Model file for the job. Use its own axes, mm. Face numbers are marked on the shaded views. A direction names the side the tool comes from. Give positions to 0.01 mm unless a question says otherwise; leave off trailing zeros. Order: outer loops, then holes, each group sorted by start corner. A loop starts at its lowest first (then second) coordinate and runs counter-clockwise, first axis right, second up. Notation, with made-up numbers: M 55.25,-28 L 103.25,-28 A30 ccw 103.25,-4 Z; hole C -36.75,42.25 d2. An arc over 180 degrees is marked long. Return JSON: item names as keys, results as strings. Group by question number.
1. Wall check: probe 1 along Y at (x, z) = (23.5, 6.75); probe 2 along Y at (x, z) = (102, 4.5); probe 3 along Y at (x, z) = (85, 5.25). Give the ranges that are in metal, low to high. Write a range as [from, to].
2. 3-axis set-ups, long thin cutter, end or side, ignore diameter. For the marked faces 4, 5 and 6: which of +Z, -Z, +X, -X, +Y, -Y reach the whole face in a straight line?
3. Pin check, flat tips, straight feed: pin 1 (15 mm diameter, centred on x = 26.5, y = 30.5, fed in from -Z) (3 decimals); pin 2 (2 mm diameter, centred on y = 60, z = 21, fed in from +X); pin 3 (5 mm diameter, centred on x = 111, y = 57, fed in from +Z). Stop position of each tip, or through.
4. Slice it at D-D on y = 16.5. List the corners of the cut face in (x, z) (3 decimals).
5. Slice it at B-B on y = 33.5. List the corners of the cut face in (x, z) (3 decimals), then the cut area to 3 significant figures.
6. Two-plate mould, pull along Y, no slides. Class the marked faces 1, 2 and 3: released by +Y, released by -Y, zero draft, split by the parting line, or undercut.
7. Slice it at C-C on x = 27.5. List the corners of the cut face in (y, z) (3 decimals).
8. Slice it at A-A on z = 5.5. List the corners of the cut face in (x, y) (3 decimals).
from build123d import *

# Parameters (mm, degrees)
F1_DEPTH = 22.225
F3_DEPTH = 19.685
F5_DEPTH = 19.685
F6_R     = 21
F6_R_2   = 18.75
F7_DEPTH = 7
F8_R     = 1.2446
F9_DEPTH = 2.541


with BuildPart() as f1:
    # F0 (on Top) → F1 (new body)
    with BuildSketch(Plane.XY):
        with BuildLine():
            ThreePointArc((0, 3.175), (0.929936, 0.929936), (3.175, 0))
            Line((3.175, 0), (88.9, 0))
            Line((88.9, 0), (88.9, 29.21))
            ThreePointArc((88.9, 29.21), (73.66, 44.45), (88.9, 59.69))
            Line((88.9, 59.69), (88.9, 88.9))
            Line((88.9, 88.9), (3.175, 88.9))
            ThreePointArc((3.175, 88.9), (0.929936, 87.970064), (0, 85.725))
            Line((0, 85.725), (0, 3.175))
        make_face()
        with BuildLine():
            Line((88.9, 29.21), (88.9, 0))
            ThreePointArc((88.9, 0), (133.35, 44.45), (88.9, 88.9))
            Line((88.9, 88.9), (88.9, 59.69))
            ThreePointArc((88.9, 59.69), (99.676307, 55.226307), (104.14, 44.45))
            ThreePointArc((104.14, 44.45), (99.676307, 33.673693), (88.9, 29.21))
        make_face()
    extrude(amount=F1_DEPTH)

    # F2 (on face) → F3 (cut)
    with BuildSketch(Plane.XY.offset(22.225)):
        with BuildLine():
            Line((88.9, 86.36), (88.9, 2.54))
            ThreePointArc((88.9, 2.54), (130.81, 44.45), (88.9, 86.36))
        make_face()
        with BuildLine():
            Line((56.642, 2.54), (88.9, 2.54))
            Line((88.9, 2.54), (88.9, 86.36))
            Line((88.9, 86.36), (56.642, 86.36))
            ThreePointArc((56.642, 86.36), (49.817005, 83.532995), (46.99, 76.708))
            Line((46.99, 76.708), (46.99, 12.192))
            ThreePointArc((46.99, 12.192), (49.817005, 5.367005), (56.642, 2.54))
        make_face()
    extrude(amount=-F3_DEPTH, mode=Mode.SUBTRACT)

    # F4 (on face) → F5 (cut)
    with BuildSketch(Plane(origin=(0, 0, 0), x_dir=(1, 0, 0), z_dir=(0, 0, -1))):
        with BuildLine():
            ThreePointArc((56.204695, -70.669557), (46.99, -44.45), (56.204695, -18.230443))
            ThreePointArc((56.204695, -18.230443), (57.376711, -8.015994), (48.674868, -2.54))
            Line((48.674868, -2.54), (2.54, -2.54))
            Line((2.54, -2.54), (2.54, -86.36))
            Line((2.54, -86.36), (48.674868, -86.36))
            ThreePointArc((48.674868, -86.36), (57.376711, -80.884006), (56.204695, -70.669557))
        make_face()
    extrude(amount=-F5_DEPTH, mode=Mode.SUBTRACT)

    # F6 (on face) → F7 (join)
    with BuildSketch(Plane.XY.offset(2.54)):
        with Locations((88.9, 44.45)):
            Circle(F6_R)
        with Locations((88.9, 44.45)):
            Circle(F6_R_2, mode=Mode.SUBTRACT)
    extrude(amount=F7_DEPTH)

    # F8 (on face) → F9 (cut, through all)
    with BuildSketch(Plane(origin=(0, 0, 19.685), x_dir=(1, 0, 0), z_dir=(0, 0, -1))):
        with Locations((10.1092, -43.18)):
            Circle(F8_R)
        with Locations((14.6304, -6.5786)):
            Circle(F8_R)
        with Locations((41.1226, -22.1996)):
            Circle(F8_R)
    extrude(amount=-F9_DEPTH, mode=Mode.SUBTRACT)


solid = f1.part
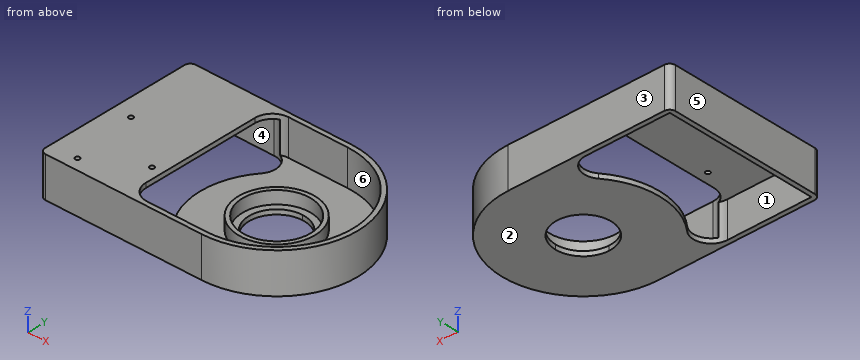
Result:
{
 "1": {"probe 1": "y = [0, 2.54], [86.36, 88.9]", "probe 2": "y = [1.97, 4.64], [28.04, 31.04], [57.86, 60.86], [84.26, 86.93]", "probe 3": "y = [0, 2.54], [23.82, 26.11], [62.79, 65.08], [86.36, 88.9]"},
 "2": {"face 4": "-Z", "face 5": "+Z, -Z, -X, +Y, -Y", "face 6": "+Z"},
 "3": {"pin 1": "stops at z = 19.685", "pin 2": "stops at x = 130.9", "pin 3": "stops at z = 2.54"},
 "4": {"outline": "M 0,0 L 2.54,0 L 2.54,19.685 L 46.99,19.685 L 46.99,22.225 L 0,22.225 Z; M 57.312,0 L 123.463,0 L 123.463,22.225 L 120.129,22.225 L 120.129,2.54 L 57.312,2.54 Z"},
 "5": {"outline": "M 0,0 L 2.54,0 L 2.54,19.685 L 46.99,19.685 L 46.99,22.225 L 0,22.225 Z; M 48.446,0 L 78.3,0 L 78.3,2.54 L 73.68,2.54 L 73.68,9.54 L 70.981,9.54 L 70.981,2.54 L 48.446,2.54 Z; M 99.5,0 L 131.98,0 L 131.98,22.225 L 129.354,22.225 L 129.354,2.54 L 106.819,2.54 L 106.819,9.54 L 104.12,9.54 L 104.12,2.54 L 99.5,2.54 Z", "area": "417 mm2"},
 "6": {"face 1": "undercut", "face 2": "zero draft", "face 3": "released by +Y"},
 "7": {"outline": "M 0,0 L 2.54,0 L 2.54,19.685 L 86.36,19.685 L 86.36,0 L 88.9,0 L 88.9,22.225 L 0,22.225 Z"},
 "8": {"outline": "M 0,3.175 A3.175 ccw 3.175,0 L 88.9,0 A44.45 ccw 88.9,88.9 L 3.175,88.9 A3.175 ccw 0,85.725 Z; C 88.9,44.45 d42; hole M 2.54,2.54 L 48.675,2.54 A9.652 ccw 52.658,3.4 A9.652 ccw 56.642,2.54 L 88.9,2.54 A41.91 ccw 88.9,86.36 L 56.642,86.36 A9.652 ccw 52.658,85.5 A9.652 ccw 48.675,86.36 L 2.54,86.36 Z; hole C 88.9,44.45 d37.5"}
}
